Build history of the part. All positions in model axes, mm. Give positions to 0.01 mm unless a question says otherwise; leave off trailing zeros. Loops run counter-clockwise (first coordinate to the right, second up) from the corner with the lowest first, then second, coordinate; pieces in that order, holes last. Notation, with made-up numbers: (54, 60.25) -> (74, 60.25) arc R17 ccw to (74, 75.25) -> close; hole circle Ø6 at (74, 46.25). An arc over 180 degrees is marked (long way). One line per question, with ' | ' between items. Start each with the question number.
(1) Slice it at A-A, the plane y = 3. Write the cut outline in (x, z), then the cut area to 3 significant figures.
(2) Mould opens along Y. For faces 1 (the face through (-0.795, -3.506, 3.493)), 2 (the face through (-0.8, -0.9, 12.27)), 3 (the face through (0, 1, 5)) say: pulls with the +Y half, pulls with the -Y half, needs draft (parallel to the pull), parting line crosses it, or undercut.
(3) Slice it at D-D, the plane z = 0.5. Write the cut outline in (x, y).
(4) Flat gauge pin, fed straight in: pin 1 Ø2 at (y, z) = (0, 15) entering from +X. Where does the tip first touch, or does it go through?
(5) Slice it at B-B, the plane y = 0.75. Write the cut outline in (x, z).
(6) Slice it at C-C, the plane x = -1.25. Write the cut outline in (y, z).
(7) Drill centre lines: L1, parallel to Z at x = -0.6, y = 1.5; L2, parallel to Z at x = -0.25, y = 1.75; L3, parallel to Y at x = -1.25, z = -5. Where is each one in solid material? Low to high. Write a range as from..to.
```python
from build123d import *

# Parameters (mm, degrees)
SKETCH1_R           = 2.35458
SKETCH1_R_2         = 2.01676
BOSS_EXTRUDE1_DEPTH = 1.6129


with BuildPart() as part:
    # Sketch1 → Boss-Extrude1 (new body)
    with BuildSketch(Plane(origin=(0, 0, 0), x_dir=(0, 0, -1), z_dir=(1, 0, 0))):
        with BuildLine():
            Line((-14.445578284, 5.64642), (5.315621716, 5.64642))
            ThreePointArc((5.315621716, 5.64642), (8.926525669, 2.385276419), (6.048845981, -1.538069657))
            Line((6.048845981, -1.538069657), (-13.304950193, -5.530011426))
            ThreePointArc((-13.304950193, -5.530011426), (-20.062820754, -0.573276417), (-14.445578284, 5.64642))
        make_face()
        with Locations((-14.445578284, 0)):
            Circle(SKETCH1_R, mode=Mode.SUBTRACT)
        with Locations((5.315621716, 2.01676)):
            Circle(SKETCH1_R_2, mode=Mode.SUBTRACT)
    extrude(amount=-BOSS_EXTRUDE1_DEPTH)


solid = part.part
```
Final values:
1) outline: (-1.61, -8.81) -> (0, -8.81) -> (0, -7.08) -> (-1.61, -7.08) -> close; (-1.61, -3.55) -> (0, -3.55) -> (0, 19.23) -> (-1.61, 19.23) -> close | area: 39.5 mm2
2) face 1: pulls with the -Y half | face 2: undercut | face 3: needs draft
3) outline: (-1.61, -2.89) -> (0, -2.89) -> (0, 5.65) -> (-1.61, 5.65) -> close
4) pin 1: through
5) outline: (-1.61, -8.72) -> (0, -8.72) -> (0, -6.88) -> (-1.61, -6.88) -> close; (-1.61, -3.75) -> (0, -3.75) -> (0, 12.21) -> (-1.61, 12.21) -> close; (-1.61, 16.68) -> (0, 16.68) -> (0, 20.04) -> (-1.61, 20.04) -> close
6) outline: (-5.53, 13.3) -> (-1.54, -6.05) arc R3.63 ccw to (5.65, -5.32) -> (5.65, 14.45) arc R5.65 ccw (long way) to start; hole circle Ø4.71 at (0, 14.45); hole circle Ø4.03 at (2.02, -5.32)
7) L1: -8.91..-7.27, -3.37..12.63, 16.26..19.89 | L2: -8.94..-7.31, -3.32..12.87, 16.02..19.81 | L3: -1.75..0.02, 4.01..5.65
